Geometry: final body of the model. Coordinates: model frame, mm. Round coordinates to 2 decimals unless told otherwise and drop trailing zeros. Write each loop counter-clockwise with the first axis right and the second up, starting at its lowest first coordinate (ties: lowest second). Pieces come first, ordered by that corner, then holes. Notation, with made-up numbers: (-24, -25.75) -> (27, -25.75) arc R16 ccw to (27, -15.75) -> close; hole circle Ø6 at (86.25, -22). An arc over 180 degrees is marked (long way). Use one line per item in the form item = value. Start each with the question number.
1. Pin query (flat end, axial travel): pin 1 Ø5 at (x, z) = (66, 61) entering from +Y. Return the tip coordinate at first contact, or that it passes through.
2. Cut plane C-C, the plane y = 0.75. State how many separate pieces and enclosed holes the cut face has, plus the area to 3 significant figures.
3. Draft query along X for faces 1 (the face through (67.56, 0.99, 69.46)), 2 (the face through (74.153, 1.014, -76.245)), 3 (the face through (67, 0, -1)). Return one class per face: pulls with the +X half, pulls with the -X half, needs draft (parallel to the pull), parting line crosses it, or undercut.
4. Cut plane B-B, the plane z = 70. Return the cut outline in (x, y).
5. Cut plane D-D, the plane x = 17. Return the cut outline in (y, z), plus the area to 3 significant figures.
6. Cut plane A-A, the plane z = -50.5. Return the cut outline in (x, y).
7. Line query: L1, parallel to X at y = 0.75, z = -61; L2, parallel to X at y = 0.7, z = -70; L3, parallel to Z at x = -8, y = 1.85. Output: solid intervals per line, ascending.
```python
from build123d import *

# Parameters (mm, degrees)
CROQUIS1_W              = 160
CROQUIS1_H              = 160
CROQUIS1_R              = 2.5
CROQUIS1_R_2            = 1.5
CROQUIS1_W_2            = 115
CROQUIS1_H_2            = 115
SALIENTE_EXTRUIR1_DEPTH = 2
CROQUIS3_W              = 170
CROQUIS3_H              = 170
CORTAR_EXTRUIR1_DEPTH   = 10


with BuildPart() as part:
    # Croquis1 → Saliente-Extruir1 (new body)
    with BuildSketch(Plane(origin=(0, 0, 0), x_dir=(1, 0, 0), z_dir=(0, 1, 0))):
        Rectangle(CROQUIS1_W, CROQUIS1_H)
        with Locations(Location((-70, 70, 0), (0, 0, 270))):
            Circle(CROQUIS1_R, mode=Mode.SUBTRACT)
        with Locations(Location((70, 70, 0), (0, 0, 270))):
            Circle(CROQUIS1_R, mode=Mode.SUBTRACT)
        with Locations(Location((70, -70, 0), (0, 0, 270))):
            Circle(CROQUIS1_R, mode=Mode.SUBTRACT)
        with Locations(Location((-70, -70, 0), (0, 0, 270))):
            Circle(CROQUIS1_R, mode=Mode.SUBTRACT)
        with Locations(Location((-61, 61, 0), (0, 0, 270))):
            Circle(CROQUIS1_R_2, mode=Mode.SUBTRACT)
        with Locations(Location((66, 61, 0), (0, 0, 270))):
            Circle(CROQUIS1_R_2, mode=Mode.SUBTRACT)
        with Locations(Location((66, -61, 0), (0, 0, 270))):
            Circle(CROQUIS1_R_2, mode=Mode.SUBTRACT)
        with Locations(Location((-61, -61, 0), (0, 0, 270))):
            Circle(CROQUIS1_R_2, mode=Mode.SUBTRACT)
        Rectangle(CROQUIS1_W_2, CROQUIS1_H_2, mode=Mode.SUBTRACT)
    extrude(amount=SALIENTE_EXTRUIR1_DEPTH)

    # Croquis3 → Cortar-Extruir1 (cut)
    with BuildSketch(Plane(origin=(0, 2, 0), x_dir=(1, 0, 0), z_dir=(0, 1, 0))):
        Rectangle(CROQUIS3_W, CROQUIS3_H)
        with BuildLine():
            Line((72.785430073, -76.963575182), (-72.785430073, -76.963575182))
            ThreePointArc((-72.785430073, -76.963575182), (-75.303300859, -75.303300859), (-76.963575182, -72.785430073))
            Line((-76.963575182, -72.785430073), (-76.963575182, 72.785430073))
            ThreePointArc((-76.963575182, 72.785430073), (-74.20471607, 76.210504229), (-70, 77.5))
            Line((-70, 77.5), (70, 77.5))
            ThreePointArc((70, 77.5), (74.20471607, 76.210504229), (76.963575182, 72.785430073))
            Line((76.963575182, 72.785430073), (76.963575182, -72.785430073))
            ThreePointArc((76.963575182, -72.785430073), (75.303300859, -75.303300859), (72.785430073, -76.963575182))
        make_face(mode=Mode.SUBTRACT)
    extrude(amount=-CORTAR_EXTRUIR1_DEPTH, mode=Mode.SUBTRACT)


solid = part.part
```
Outcome:
q1.pin_1 = 2
q2.separate_pieces = 1
q2.enclosed_holes = 9
q2.area = 10,400 mm^2
q3.face_1 = undercut
q3.face_2 = pulls with the +X half
q3.face_3 = needs draft
q4.outline = (-76.96, 0) -> (-72.5, 0) -> (-72.5, 2) -> (-76.96, 2) -> close; (-67.5, 0) -> (67.5, 0) -> (67.5, 2) -> (-67.5, 2) -> close; (72.5, 0) -> (76.96, 0) -> (76.96, 2) -> (72.5, 2) -> close
q5.outline = (0, -77.5) -> (2, -77.5) -> (2, -57.5) -> (0, -57.5) -> close; (0, 57.5) -> (2, 57.5) -> (2, 76.96) -> (0, 76.96) -> close
q5.area = 78.9 mm^2
q6.outline = (-76.96, 0) -> (-57.5, 0) -> (-57.5, 2) -> (-76.96, 2) -> close; (57.5, 0) -> (76.96, 0) -> (76.96, 2) -> (57.5, 2) -> close
q7.L1 = -76.96 to -62.5, -59.5 to 64.5, 67.5 to 76.96
q7.L2 = -76.96 to -72.5, -67.5 to 67.5, 72.5 to 76.96
q7.L3 = -77.5 to -57.5, 57.5 to 76.96
